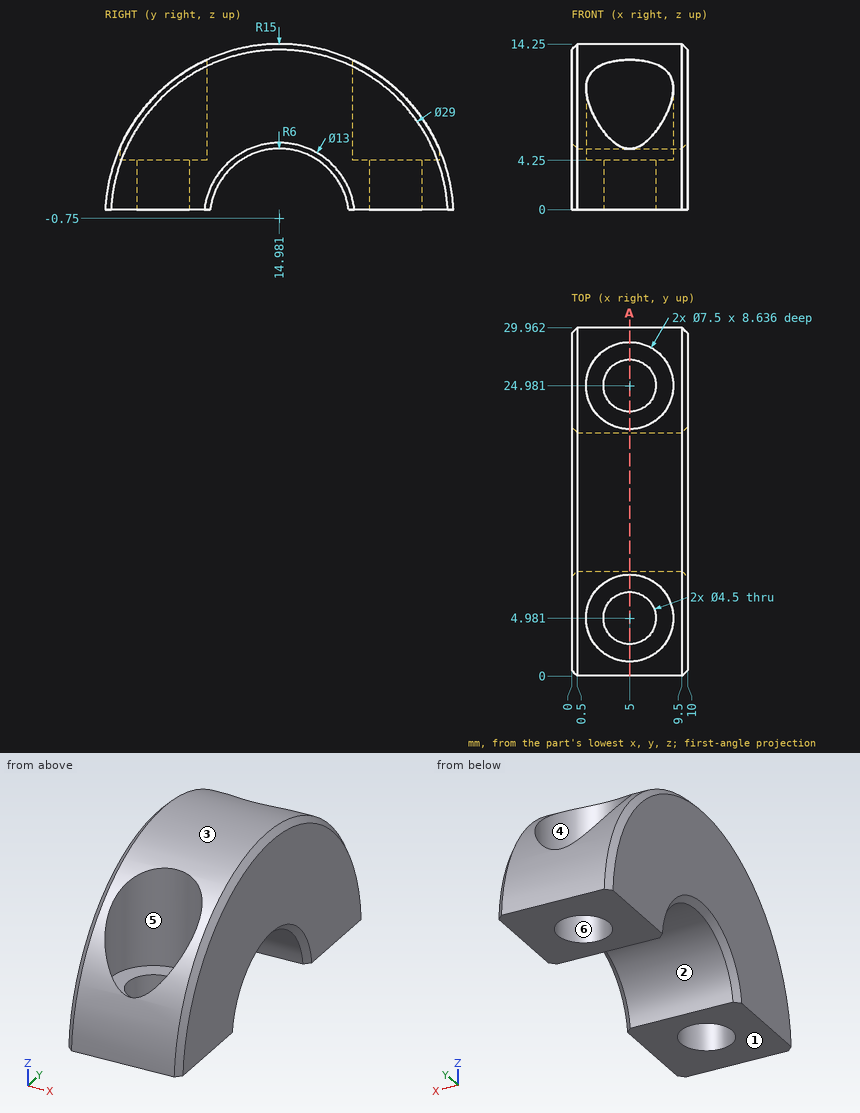
Geometry: see drawing. Coordinates: mm, zero at the bounding-box minimum. A direction names the side the tool comes from. Give positions to 0.01 mm unless a question says otherwise; leave off trailing zeros. Answer in a Markdown table with one row per item. Add a question column.
(1) Ray query, line 1 (X direction, y = 27.25, z = 5.25) (1 decimal); line 2 (Z direction, x = 7.25, y = 6.5); line 3 (X direction, y = 6.5, z = 9). Return the intervals inside material, ascending.
(2) Mould query, pull axis Y, two halves, no side actions, for the marked faces 1, 2, 3 and 4. Classes: +Y half, -Y half, draft (parallel to the pull), parting line (faces both ways), or undercut.
(3) First-contact query: pin 1 (6 mm diameter, centred on x = 4.5, y = 23.5, fed in from +Z). Flat tip, straight axial feed; report the tip coordinate or a pass-through.
(4) Reachability of the marked faces 5 and 6 from +Z, -Z, +X, -X, +Y, -Y: full face, straight path, thin tool, end or side. Return the list, or none.
(5) Section A-A on x = 5. State how many separate pieces and enclosed holes the cut face has, and give its area (3 significant figures).
Result set:
| question | item | result |
|---|---|---|
| 1 | line 1 | x = 0 to 2, 8 to 10 |
| 1 | line 2 | z = 0 to 4.25 |
| 1 | line 3 | x = 0 to 1.57, 8.43 to 10 |
| 2 | face 1 | draft |
| 2 | face 2 | undercut |
| 2 | face 3 | parting line |
| 2 | face 4 | undercut |
| 3 | pin 1 | stops at z = 13.2 |
| 4 | face 5 | +Z |
| 4 | face 6 | +Z, -Z |
| 5 | separate pieces | 3 |
| 5 | enclosed holes | 0 |
| 5 | area | 159 mm^2 |
